The listing builds one solid part. Answer for the finished solid, in the listing's coordinates (mm). A direction names the side the tool comes from. Give positions to 0.01 mm unless a question says otherwise; leave off trailing zeros. Order: outer loops, then holes, each group sorted by start corner. A loop starts at its lowest first (then second) coordinate and runs counter-clockwise, first axis right, second up.
```python
from build123d import *

# Parameters (mm, degrees)
F1_W     = 50
F1_H     = 100
F2_DEPTH = 935
F3_W     = 100
F3_H     = 30
F4_DEPTH = 100.001


with BuildPart() as f2:
    # F1 (on Right) → F2 (new body, symmetric)
    with BuildSketch(Plane.YZ):
        Rectangle(F1_W, F1_H)
    extrude(amount=F2_DEPTH, both=True)

    # F3 (on face) → F4 (cut, through all)
    with BuildSketch(Plane.XY.offset(50)):
        with Locations((-885, 10)):
            Rectangle(F3_W, F3_H)
        with Locations((885, 10)):
            Rectangle(F3_W, F3_H)
    extrude(amount=-F4_DEPTH, mode=Mode.SUBTRACT)


solid = f2.part
```
1) Find section A-A (z = 17.5). Write down the section's boundary in (x, y).
Geometry says:
outline: (-935, -25) - (935, -25) - (935, -5) - (835, -5) - (835, 25) - (-835, 25) - (-835, -5) - (-935, -5) - close
2) A tool of negligible diameter and unlimited length cuts with its end or side. For faces 1 (the flat face through (-886, -5, 1)), 2 (the flat face through (13, -25, -1)), 3 (the flat face through (884, -5, 1)), from which of +Z, -Z, +X, -X, +Y, -Y can it reach the whole face along a straight path? Write none if from no direction.
Geometry says:
face 1: +Z, -Z, -X, +Y
face 2: +Z, -Z, +X, -X, -Y
face 3: +Z, -Z, +X, +Y
3) Find section B-B (y = 4). Write down the section's boundary in (x, z), then the cut area to 3 significant figures.
Geometry says:
outline: (-835, -50) - (835, -50) - (835, 50) - (-835, 50) - close
area: 167,000 mm2
4) Given P1, Ø15, axis at y = 12.5, z = -9, coming from the +X side; P2, Ø9, axis at y = 8.5, z = 3, coming from the -X side, each flat-ended and moving along its own axis, determine where each tip first touches the part or whether it passes through.
Geometry says:
P1: stops at x = 835
P2: stops at x = -835
5) Straight lines are drawn through the part: probe 1 along Y at (x, z) = (-855.5, 44.5); probe 2 along X at (y, z) = (12.5, 11). For each, find the intervals that lie inside material, in ascending order.
Geometry says:
probe 1: y = -25 to -5
probe 2: x = -835 to 835
